```python
from build123d import *

# Parameters (mm, degrees)
BOSS_EXTRUDE2_DEPTH = 50
BOSS_EXTRUDE3_DEPTH = 20
BOSS_EXTRUDE4_DEPTH = 7.5
FILLET2_R           = 20
FILLET3_R           = 20


with BuildPart() as part:
    # Sketch2 → Boss-Extrude2 (new body)
    with BuildSketch(Plane(origin=(0, 0, 0), x_dir=(0, 0, -1), z_dir=(1, 0, 0))):
        Polygon((0, 0), (25, 0), (25, 20), (20, 20), (20, 10), (10, 10), (10, 80), (0, 80), align=None)
    extrude(amount=BOSS_EXTRUDE2_DEPTH)

    # Sketch3 → Boss-Extrude3 (add)
    with BuildSketch(Plane(origin=(0, 70, 0), x_dir=(1, 0, 0), z_dir=(0, 1, 0))):
        Polygon((50, 0), (60, 0), (60, 25), (45, 25), (45, 20), (50, 20), (55, 20), (55, 10), (50, 10), align=None)
    boss_extrude3 = extrude(amount=-BOSS_EXTRUDE3_DEPTH)

    # Mirror1: Boss-Extrude3 across plane
    add(boss_extrude3.mirror(Plane(origin=(25, 0, 0), x_dir=(0, 0, 1), z_dir=(1, 0, 0))))

    # Sketch5 → Boss-Extrude4 (add, symmetric)
    with BuildSketch(Plane(origin=(25, 0, 0), x_dir=(0, 0, -1), z_dir=(1, 0, 0))):
        Polygon((0, 80), (-38.670604871, 80), (-103.005812487, 50), (-103.005812487, 0), (-80.902994242, 0), (-63.207021205, 8.251767746), (-67.433203822, 17.314845616), (-85.559359563, 8.862480381), (-90.630778704, 19.738173826), (0, 62), align=None)
    extrude(amount=BOSS_EXTRUDE4_DEPTH, both=True)

    # Fillet2
    fillet2_edges = [part.edges().sort_by_distance(p)[0] for p in [
        (25, 80, 38.670604871),
    ]]
    fillet(fillet2_edges, radius=FILLET2_R)

    # Fillet3
    fillet3_edges = [part.edges().sort_by_distance(p)[0] for p in [
        (25, 50, 103.005812487),
    ]]
    fillet(fillet3_edges, radius=FILLET3_R)


solid = part.part
```
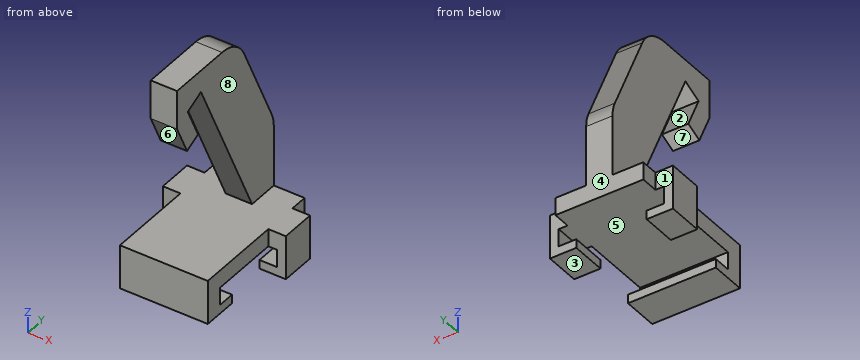
Input: part model. Units: mm. Frame: model coordinates. Face numbers are marked on the shaded views. A direction names the side the tool comes from. Coordinates: 2 decimals unless noted, no trailing zeros. Loops run counter-clockwise (first coordinate to the right, second up) from the corner with the lowest first, then second, coordinate; pieces in that order, holes last. Notation, with made-up numbers: M 78,36 L 86,36 A26 ccw 86,75 Z; hole C -37,15 d4. An arc over 180 degrees is marked long. Use a Markdown table: item, result. Add a question column.
1) Draft query along Y for the marked faces 1, 2 and 3. Return one class per face: +Y half, -Y half, draft (parallel to the pull), parting line (faces both ways), or undercut.
2) Section B-B, the plane z = -17. Return the cut outline in (x, y).
3) Pin query (flat end, axial travel): P1, Ø5, axis at x = 50.5, y = 60.5, coming from the +Z side; P2, Ø1.5, axis at x = 32.5, y = 59.5, coming from the -Z side; P3, Ø4.5, axis at x = -1.5, z = -10.5, coming from the -Y side; P4, Ø10, axis at y = 45.5, z = 62.5, coming from the +X side. Return the tip coordinate at first contact, or that it passes through.
4) Set-up query: the marked faces 4, 5, 6, 7 and 8. Return all of +Z, -Z, +X, -X, +Y, -Y with unobstructed straight access to the full face (end or side cutting, diameter ignored); none if empty.
5) Section D-D, the plane z = 65.5. Return the cut outline in (x, y).
6) Section A-A, the plane x = 47. Return the cut outline in (y, z).
7) Section C-C, the plane y = 26. Return the cut outline in (x, z).
8) Line query: L1, parallel to Z at x = 53.5, y = 57; L2, parallel to X at y = 66.5, z = -16.5; L3, parallel to Z at x = 16, y = 44.5. Output: solid intervals per line, ascending. Write a range as from..to.
Answer below:
| question | item | result |
|---|---|---|
| 1 | face 1 | +Y half |
| 1 | face 2 | undercut |
| 1 | face 3 | draft |
| 2 | outline | M -10,50 L -5,50 L -5,70 L -10,70 Z; M 0,0 L 50,0 L 50,10 L 0,10 Z; M 55,50 L 60,50 L 60,70 L 55,70 Z |
| 3 | P1 | z = 0 |
| 3 | P2 | z = -10 |
| 3 | P3 | y = 0 |
| 3 | P4 | x = 32.5 |
| 4 | face 4 | +Z, -Z, +X, -X, +Y |
| 4 | face 5 | +Y |
| 4 | face 6 | +X, -X, -Y |
| 4 | face 7 | +X, -X |
| 4 | face 8 | +Z, +X, +Y, -Y |
| 5 | outline | M 17.5,7.18 L 32.5,7.18 L 32.5,13.17 L 17.5,13.17 Z; M 17.5,31.46 L 32.5,31.46 L 32.5,67.49 L 17.5,67.49 Z |
| 6 | outline | M 0,-25 L 20,-25 L 20,-20 L 10,-20 L 10,-10 L 80,-10 L 80,0 L 0,0 Z; M 50,-25 L 70,-25 L 70,-20 L 50,-20 Z |
| 7 | outline | M 0,-10 L 50,-10 L 50,0 L 0,0 Z; M 17.5,77.2 L 32.5,77.2 L 32.5,103.01 L 17.5,103.01 Z |
| 8 | L1 | -25..-20, -10..0 |
| 8 | L2 | -10..-5, 55..60 |
| 8 | L3 | -10..0 |
